```python
from build123d import *

# Parameters (mm, degrees)
BOSS_EXTRUDE1_DEPTH = 11.90625
SKETCH2_W           = 6.35
SKETCH2_H           = 28.575
CUT_EXTRUDE1_DEPTH  = 12.90625


with BuildPart() as part:
    # Sketch1 → Boss-Extrude1 (new body)
    with BuildSketch(Plane.XY):
        Polygon((-284.234659091, -116.031818182), (-284.234659091, -712.931818182), (-165.965909091, -712.931818182), (-165.965909091, -916.131818182), (407.915340909, -916.131818182), (407.915340909, 296.718181818), (114.227840909, 296.718181818), align=None)
    extrude(amount=BOSS_EXTRUDE1_DEPTH)

    # Sketch2 → Cut-Extrude1 (cut, through all)
    with BuildSketch(Plane.XY.offset(11.90625)):
        with Locations((-281.059659091, -586.693818182)):
            Rectangle(SKETCH2_W, SKETCH2_H)
        with Locations((-281.059659091, -446.993818182)):
            Rectangle(SKETCH2_W, SKETCH2_H)
        with Locations((-281.059659091, -307.293818182)):
            Rectangle(SKETCH2_W, SKETCH2_H)
    extrude(amount=-CUT_EXTRUDE1_DEPTH, mode=Mode.SUBTRACT)


solid = part.part
```
Input: part model. Units: mm. Frame: model coordinates. Give positions to 0.01 mm unless a question says otherwise; leave off trailing zeros. Order: outer loops, then holes, each group sorted by start corner. A loop starts at its lowest first (then second) coordinate and runs counter-clockwise, first axis right, second up. Notation, with made-up numbers: M 76,21 L 99,21 A19 cw 99,38 Z; hole C 16,-19 d7. An arc over 180 degrees is marked long. Return JSON: item names as keys, results as strings.
1) Line query: L1, parallel to X at y = -713, z = 2.5; L2, parallel to Y at x = -116, z = 5.5; L3, parallel to Y at x = 39.5, z = 8.5. Output: solid intervals per line, ascending. Write a range as [from, to].
Taken from the geometry:
{"L1": "x = [-165.97, 407.92]", "L2": "y = [-916.13, 58.24]", "L3": "y = [-916.13, 219.31]"}
2) Contact query for flat-ended pins moving along their axis: pin 1 (5 mm diameter, centred on x = -281, z = 6.5, fed in from -Y); pin 2 (3.5 mm diameter, centred on y = -312, z = 5, fed in from -X); pin 3 (3 mm diameter, centred on x = -281, z = 5, fed in from +Y). Output: stop coordinate, or through.
Taken from the geometry:
{"pin 1": "stops at y = -712.93", "pin 2": "stops at x = -277.88", "pin 3": "stops at y = -111.13"}
3) Section query B-B on x = 62. Output: boundary loops of the cut face in (y, z), and give its area (3 significant figures).
Taken from the geometry:
{"outline": "M -916.13,0 L 242.62,0 L 242.62,11.91 L -916.13,11.91 Z", "area": "13,800 mm2"}
4) Section query A-A on z = 3.5. Output: boundary loops of the cut face in (x, y), and give its area (3 significant figures).
Taken from the geometry:
{"outline": "M -284.23,-712.93 L -165.97,-712.93 L -165.97,-916.13 L 407.92,-916.13 L 407.92,296.72 L 114.23,296.72 L -284.23,-116.03 L -284.23,-293.01 L -277.88,-293.01 L -277.88,-321.58 L -284.23,-321.58 L -284.23,-432.71 L -277.88,-432.71 L -277.88,-461.28 L -284.23,-461.28 L -284.23,-572.41 L -277.88,-572.41 L -277.88,-600.98 L -284.23,-600.98 Z", "area": "733,000 mm2"}
5) Section query C-C on y = 197. Output: boundary loops of the cut face in (x, z), and give its area (3 significant figures).
Taken from the geometry:
{"outline": "M 17.96,0 L 407.92,0 L 407.92,11.91 L 17.96,11.91 Z", "area": "4,640 mm2"}
